```python
from build123d import *

# Parameters (mm, degrees)
BOSS_EXTRUDE3_DEPTH = 8
SKETCH4_R           = 2
CUT_EXTRUDE3_DEPTH  = 14.285330256


with BuildPart() as part:
    # Sketch3 → Boss-Extrude3 (new body)
    with BuildSketch(Plane.XY):
        Polygon((7.5, 0), (3.09302731, 0), (0, 0), (0, -0.8), (7.5, -0.8), align=None)
        Polygon((4.40697269, 5.9), (7.5, 5.9), (3.09302731, 4.72), (7.5, 3.54), (3.09302731, 2.36), (7.5, 1.18), (3.09302731, 0), (0, 0), (4.40697269, 1.18), (0, 2.36), (4.40697269, 3.54), (0, 4.72), align=None)
        Polygon((4.40697269, 5.9), (7.5, 5.9), (7.5, 6.7), (0, 6.7), (0, 5.9), align=None)
    extrude(amount=BOSS_EXTRUDE3_DEPTH)

    # Sketch4 → Cut-Extrude3 (cut, through all)
    with BuildSketch(Plane.XZ.offset(0.8)):
        with Locations(Location((3.75, 4, 0), (0, 0, 270))):
            Circle(SKETCH4_R)
    extrude(amount=-CUT_EXTRUDE3_DEPTH, mode=Mode.SUBTRACT)


solid = part.part
```
Input: part model. Units: mm. Frame: model coordinates. Round coordinates to 2 decimals unless told otherwise and drop trailing zeros. Loops run counter-clockwise (first coordinate to the right, second up) from the corner with the lowest first, then second, coordinate; pieces in that order, holes last. Notation, with made-up numbers: (35.5, 51.25) -> (43.5, 51.25) arc R20 ccw to (43.5, 69.25) -> close; hole circle Ø3 at (48.25, 83.5). An arc over 180 degrees is marked (long way). Use one line per item in the form item = value. Start each with the question number.
Item 1: Section query C-C on y = 6.25. Return the cut outline in (x, z), then the cut area to 3 significant figures.
Item 2: Section query D-D on x = 7. Return the cut outline in (y, z), then the cut area to 3 significant figures.
Item 3: Section query A-A on z = 3. Return the cut outline in (x, y).
Item 4: Section query B-B on x = 5. Count the separate pieces of the cut face and the enclosed holes in it, then the cut area to 3 significant figures.
Item 5: Contact query for a flat-ended pin moving along its axis: pin 1 Ø1 at (y, z) = (2, 3.5) entering from -X. Output: stop coordinate, or through.
Item 6: Mould query, pull axis Y, two halves, no side actions, for faces 1 (the face through (4, 3, 0)), 2 (the face through (6.245, 3.876, 3.944)), 3 (the face through (5, 6.7, 2)), 4 (the face through (6.31, 3.22, 3.94)). Classes: pulls with the +Y half, pulls with the -Y half, needs draft (parallel to the pull), parting line crosses it, or undercut.
Item 7: Material intervals for L1, parallel to Y at x = 1.25, z = 2.25; L2, parallel to Y at x = 1, z = 0.5; L3, parallel to Z at x = 3.75, y = 4.5, sorted ascending. Write a range as from..to.
Ans:
q1.outline = (0, 0) -> (7.5, 0) -> (7.5, 8) -> (0, 8) -> close; hole circle Ø4 at (3.75, 4)
q1.area = 47.4 mm^2
q2.outline = (-0.8, 0) -> (0, 0) -> (0, 8) -> (-0.8, 8) -> close; (1.05, 0) -> (1.31, 0) -> (1.31, 8) -> (1.05, 8) -> close; (3.41, 0) -> (3.67, 0) -> (3.67, 8) -> (3.41, 8) -> close; (5.77, 0) -> (6.7, 0) -> (6.7, 8) -> (5.77, 8) -> close
q2.area = 18.2 mm^2
q3.outline = (0, -0.8) -> (2.02, -0.8) -> (2.02, 0.54) -> (0, 0) -> close; (0, 2.36) -> (2.02, 1.82) -> (2.02, 2.9) -> close; (0, 4.72) -> (2.02, 4.18) -> (2.02, 5.26) -> close; (0, 5.9) -> (2.02, 5.9) -> (2.02, 6.7) -> (0, 6.7) -> close; (5.48, -0.8) -> (7.5, -0.8) -> (7.5, 0) -> (5.48, 0) -> close; (5.48, 0.64) -> (7.5, 1.18) -> (5.48, 1.72) -> close; (5.48, 3) -> (7.5, 3.54) -> (5.48, 4.08) -> close; (5.48, 5.36) -> (7.5, 5.9) -> (7.5, 6.7) -> (5.48, 6.7) -> close
q4.separate_pieces = 8
q4.enclosed_holes = 0
q4.area = 24.1 mm^2
q5.pin_1 = 0
q6.face_1 = needs draft
q6.face_2 = undercut
q6.face_3 = pulls with the +Y half
q6.face_4 = undercut
q7.L1 = -0.8..0.33, 2.03..2.69, 4.39..5.05, 5.9..6.7
q7.L2 = -0.8..0.27, 2.09..2.63, 4.45..4.99, 5.9..6.7
q7.L3 = 0..2, 6..8
